```python
from build123d import *

# Parameters (mm, degrees)
F0_R     = 10
F1_DEPTH = 6
F2_DEPTH = 26
F3_DEPTH = 20


with BuildPart() as f1:
    # F0 (on Top) → F1 (new body)
    with BuildSketch(Plane.XY):
        with BuildLine():
            Line((-6, -17.5), (0, -17.5))
            ThreePointArc((0, -17.5), (17.5, 0), (0, 17.5))
            Line((0, 17.5), (-35, 17.5))
            ThreePointArc((-35, 17.5), (-15.938437, 3.77958), (-6, -17.5))
        make_face()
        Circle(F0_R, mode=Mode.SUBTRACT)
        with BuildLine():
            Line((-180, -17.5), (-6, -17.5))
            ThreePointArc((-6, -17.5), (-15.938437, 3.77958), (-35, 17.5))
            Line((-35, 17.5), (-155, 17.5))
            Line((-155, 17.5), (-165, 67.5))
            Line((-165, 67.5), (-190, 67.5))
            Line((-190, 67.5), (-190, -7.5))
            ThreePointArc((-190, -7.5), (-187.071068, -14.571068), (-180, -17.5))
        make_face()
        with Locations((-85, 0)):
            Circle(F0_R, mode=Mode.SUBTRACT)
        with BuildLine():
            Line((-190, 67.5), (-165, 67.5))
            Line((-165, 67.5), (-170.072186, 69.528875))
            ThreePointArc((-170.072186, 69.528875), (-177.5, 70.959341), (-184.927814, 69.528875))
            Line((-184.927814, 69.528875), (-190, 67.5))
        make_face()
    extrude(amount=-F1_DEPTH)

    # F0 (on Top) → F2 (join)
    with BuildSketch(Plane.XY):
        with BuildLine():
            Line((-6, -17.5), (0, -17.5))
            ThreePointArc((0, -17.5), (17.5, 0), (0, 17.5))
            Line((0, 17.5), (-35, 17.5))
            ThreePointArc((-35, 17.5), (-15.938437, 3.77958), (-6, -17.5))
        make_face()
        Circle(F0_R, mode=Mode.SUBTRACT)
        with BuildLine():
            Line((-180, -17.5), (-6, -17.5))
            ThreePointArc((-6, -17.5), (-15.938437, 3.77958), (-35, 17.5))
            Line((-35, 17.5), (-155, 17.5))
            Line((-155, 17.5), (-165, 67.5))
            Line((-165, 67.5), (-190, 67.5))
            Line((-190, 67.5), (-190, -7.5))
            ThreePointArc((-190, -7.5), (-187.071068, -14.571068), (-180, -17.5))
        make_face()
        with Locations((-85, 0)):
            Circle(F0_R, mode=Mode.SUBTRACT)
        with BuildLine():
            Line((-190, 67.5), (-165, 67.5))
            Line((-165, 67.5), (-170.072186, 69.528875))
            ThreePointArc((-170.072186, 69.528875), (-177.5, 70.959341), (-184.927814, 69.528875))
            Line((-184.927814, 69.528875), (-190, 67.5))
        make_face()
    extrude(amount=F2_DEPTH)

    # F0 (on Top) → F3 (cut)
    with BuildSketch(Plane.XY):
        with BuildLine():
            Line((-6, -17.5), (0, -17.5))
            ThreePointArc((0, -17.5), (17.5, 0), (0, 17.5))
            Line((0, 17.5), (-35, 17.5))
            ThreePointArc((-35, 17.5), (-15.938437, 3.77958), (-6, -17.5))
        make_face()
        Circle(F0_R, mode=Mode.SUBTRACT)
    extrude(amount=F3_DEPTH, mode=Mode.SUBTRACT)


solid = f1.part
```
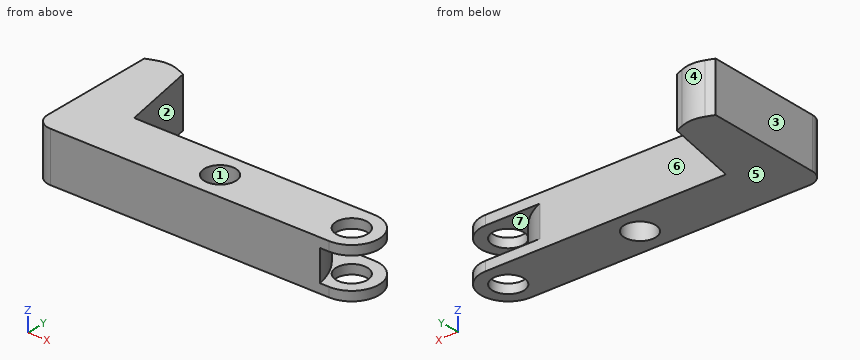
Model file for the job. Use its own axes, mm. Face numbers are marked on the shaded views. A direction names the side the tool comes from. Round coordinates to 2 decimals unless told otherwise and drop trailing zeros. Order: outer loops, then holes, each group sorted by start corner. A loop starts at its lowest first (then second) coordinate and runs counter-clockwise, first axis right, second up. Notation, with made-up numbers: (61.25, 37.5) -> (85.25, 37.5) arc R13 cw to (85.25, 51.5) -> close; hole circle Ø11 at (8.25, 26). An arc over 180 degrees is marked (long way). Use one line per item in the form item = value.
Item 1: Cut at B-B, the plane x = -85. Write the cut outline in (y, z), and give its area (3 significant figures).
Returned:
outline = (-17.5, -6) -> (-10, -6) -> (-10, 26) -> (-17.5, 26) -> close; (10, -6) -> (17.5, -6) -> (17.5, 26) -> (10, 26) -> close
area = 480 mm^2
Item 2: Tool access for the marked faces 5, 6 and 7: list every direction of +Z, -Z, +X, -X, +Y, -Y with a clear straight run to the whole face (end or side of a thin tool).
Returned:
face_5 = -Z, +X, -X, +Y, -Y
face_6 = +Z, -Z, +X, +Y
face_7 = +X, +Y
Item 3: Flat gauge pins, fed straight in: pin 1 Ø6 at (x, z) = (-123.5, 6.5) entering from +Y; pin 2 Ø18 at (x, y) = (0, 0) entering from +Z. Where does each tip first touch, or does it go through?
Returned:
pin_1 = 17.5
pin_2 = through
Item 4: Cut at C-C, the plane y = 0. Write the cut outline in (x, z), and give its area (3 significant figures).
Returned:
outline = (-190, -6) -> (-95, -6) -> (-95, 26) -> (-190, 26) -> close; (-75, -6) -> (-10, -6) -> (-10, 0) -> (-13.12, 0) -> (-13.12, 20) -> (-10, 20) -> (-10, 26) -> (-75, 26) -> close; (10, -6) -> (17.5, -6) -> (17.5, 0) -> (10, 0) -> close; (10, 20) -> (17.5, 20) -> (17.5, 26) -> (10, 26) -> close
area = 5,150 mm^2
Item 5: Cut at A-A, the plane z = 23.5. Write the cut outline in (x, y), and give its area (3 significant figures).
Returned:
outline = (-190, -7.5) arc R10 ccw to (-180, -17.5) -> (0, -17.5) arc R17.5 ccw to (0, 17.5) -> (-155, 17.5) -> (-165, 67.5) -> (-170.07, 69.53) arc R20 ccw to (-184.93, 69.53) -> (-190, 67.5) -> close; hole circle Ø20 at (-85, 0); hole circle Ø20 at (0, 0)
area = 8,040 mm^2
Item 6: Pull direction X, two halves, no side cores. Call the marked faces 1, 2, 3 and 4: released by +X, released by -X, zero draft, split by the parting line, or undercut.
Returned:
face_1 = undercut
face_2 = released by +X
face_3 = released by -X
face_4 = split by the parting line
Item 7: Cut at D-D, the plane y = 49.5. Write the cut outline in (x, z), and give its area (3 significant figures).
Returned:
outline = (-190, -6) -> (-161.4, -6) -> (-161.4, 26) -> (-190, 26) -> close
area = 915 mm^2
Item 8: Drill centre lines: line 1 (Y direction, x = -85, z = 1.5); line 2 (Y direction, x = -133.5, z = 8.5); line 3 (Y direction, x = -82.5, z = 16.5). Where is each one in solid material? Low to high.
Returned:
line_1 = -17.5 to -10, 10 to 17.5
line_2 = -17.5 to 17.5
line_3 = -17.5 to -9.68, 9.68 to 17.5
